Source: CAD feature listing. Evaluate the final solid. Frame: model axes, mm. A direction names the side the tool comes from. Give positions to 0.01 mm unless a question says otherwise; leave off trailing zeros. Write each loop counter-clockwise with the first axis right and the second up, starting at its lowest first coordinate (ties: lowest second). Pieces come first, ordered by that corner, then holes. Notation, with made-up numbers: (-22.75, 80.25) -> (30.25, 80.25) arc R13 ccw to (30.25, 99.25) -> close; hole circle Ø3 at (-32.75, -18.5). An arc over 180 degrees is marked (long way). Write item = value, one per line.
Autodesk Inventor part; units mm, degrees
ref_plane "YZ Plane" through (0, 0, 0) normal (1, 0, 0) x (0, 1, 0)
ref_plane "XZ Plane" through (0, 0, 0) normal (0, 1, 0) x (-1, 0, 0)
ref_plane "XY Plane" through (0, 0, 0) normal (0, 0, 1) x (1, 0, 0)
sketch "Эскиз1" plane through (0, 0, 0) normal (0, 0, 1) x (1, 0, 0)
  line L0 (0, 0) -> (58, 0)
  line L1 (58, 0) -> (58, 60)
  line L2 (58, 60) -> (0, 60)
  line L3 (0, 60) -> (0, 0)
  line L4 (0, 57) -> (58, 57) construction
  line L5 (0, 3) -> (58, 3) construction
  line L6 (3, 0) -> (3, 60) construction
  line L7 (55, 60) -> (55, 0) construction
  circle A0 centre (3, 57) radius 1.25
  circle A1 centre (55, 57) radius 1.25
  circle A2 centre (55, 3) radius 1.25
  circle A3 centre (3, 3) radius 1.25
  dimension "d0" = 58
  dimension "d1" = 60
  dimension "d2" = 52
  dimension "d3" = 54
  dimension "d4" = 3
  dimension "d5" = 3
  dimension "d6" = 2.5
extrude "Выдавливание1" add sketch "Эскиз1" along normal blind 1
sketch "Эскиз2" plane through (0, 0, 1) normal (0, 0, 1) x (1, 0, 0)
  line L0 (37, -2) -> (47, -2)
  line L1 (47, -2) -> (47, 10)
  line L2 (47, 10) -> (37, 10)
  line L3 (37, 10) -> (37, -2)
  line L4 (0, 60) -> (0, 0)
  line L5 (58, 0) -> (58, 60)
  line L6 (0, 0) -> (58, 0)
  dimension "d9" = 37
  dimension "d10" = 11
  dimension "d14" = 2
  dimension "d15" = 12
extrude "Выдавливание2" add sketch "Эскиз2" along normal blind 11
sketch "Эскиз3" plane through (0, 0, 1) normal (0, 0, 1) x (1, 0, 0)
  line L0 (7, 60) -> (19.5, 60)
  line L1 (19.5, 60) -> (19.5, 53)
  line L2 (19.5, 53) -> (7, 53)
  line L3 (7, 53) -> (7, 60)
  line L4 (58, 60) -> (0, 60)
  line L5 (0, 60) -> (0, 0)
  line L6 (58, 0) -> (58, 60)
  line L7 (30.5, 60) -> (43, 60)
  line L8 (43, 60) -> (43, 53)
  line L9 (43, 53) -> (30.5, 53)
  line L10 (30.5, 53) -> (30.5, 60)
  dimension "d16" = 7
  dimension "d18" = 15
  dimension "d19" = 12.5
  dimension "d20" = 7
extrude "Выдавливание3" add sketch "Эскиз3" along normal blind 6
sketch "Эскиз4" plane through (0, 0, 1) normal (0, 0, 1) x (1, 0, 0)
  line L0 (3, 50) -> (47, 50)
  line L1 (47, 50) -> (47, 35)
  line L2 (47, 35) -> (3, 35)
  line L3 (3, 35) -> (3, 50)
  line L4 (0, 60) -> (0, 0)
  line L5 (30.5, 60) -> (19.5, 60)
  dimension "d23" = 15
  dimension "d24" = 44
  dimension "d25" = 3
  dimension "d26" = 10
extrude "Выдавливание4" add sketch "Эскиз4" along normal blind 26
sketch "Эскиз5" plane through (0, 0, 1) normal (0, 0, 1) x (1, 0, 0)
  line L0 (3, 33) -> (46, 33)
  line L1 (46, 33) -> (46, 15)
  line L2 (46, 15) -> (3, 15)
  line L3 (3, 15) -> (3, 33)
  line L4 (0, 0) -> (37, 0)
  line L5 (0, 60) -> (0, 0)
  line L6 (58, 0) -> (58, 60)
  dimension "d29" = 15
  dimension "d30" = 3
  dimension "d31" = 18
  dimension "d32" = 12
extrude "Выдавливание5" add sketch "Эскиз5" along normal blind 17
sketch "Эскиз6" plane through (0, 0, 1) normal (0, 0, 1) x (1, 0, 0)
  line L0 (24, 12) -> (3, 12)
  line L1 (3, 12) -> (3, 6)
  line L2 (3, 6) -> (24, 6)
  line L3 (24, 6) -> (24, 12)
  line L4 (0, 0) -> (37, 0)
  line L5 (0, 60) -> (0, 0)
  dimension "d35" = 6
  dimension "d36" = 3
  dimension "d37" = 6
  dimension "d38" = 21
extrude "Выдавливание6" add sketch "Эскиз6" along normal blind 11
properties part number "Плата"
(1) Section query A-A (y = 3). Return loops of the section in (x, z), plus the area to 3 significant figures.
Values follow:
outline = (0, 0) -> (1.75, 0) -> (1.75, 1) -> (0, 1) -> close; (4.25, 0) -> (53.75, 0) -> (53.75, 1) -> (47, 1) -> (47, 12) -> (37, 12) -> (37, 1) -> (4.25, 1) -> close; (56.25, 0) -> (58, 0) -> (58, 1) -> (56.25, 1) -> close
area = 163 mm2
(2) Material intervals for line 1 (Y direction, x = 14, z = 1.5); line 2 (Y direction, x = 3, z = 0.4); line 3 (Y direction, x = 17, z = 9), sorted ascending.
Values follow:
line_1 = 6 to 12, 15 to 33, 35 to 50, 53 to 60
line_2 = 0 to 1.75, 4.25 to 55.75, 58.25 to 60
line_3 = 6 to 12, 15 to 33, 35 to 50
(3) First-contact query: pin 1 (5 mm diameter, centred on y = 8, z = 4, fed in from +X); pin 2 (12 mm diameter, centred on y = 34.5, z = 17.5, fed in from -X); pin 3 (2 mm diameter, centred on x = 39.5, z = 18, fed in from +Y); pin 4 (3 mm diameter, centred on x = 27, y = 7.5, fed in from -Z). Flat tips, straight axial feed; report the tip coordinate or a pass-through.
Values follow:
pin_1 = 47
pin_2 = 3
pin_3 = 50
pin_4 = 0
(4) Pull-direction query (Y, two-part tool) for faces 1 (the face through (42, -2, 6)), 2 (the face through (19.5, 57, 4)), 3 (the face through (56.19, 56.62, 0.49)); classes: pulls with the +Y half, pulls with the -Y half, needs draft (parallel to the pull), parting line crosses it, or undercut.
Values follow:
face_1 = pulls with the -Y half
face_2 = needs draft
face_3 = undercut
(5) Access query for faces 4 (the face through (37, 4, 6)), 5 (the face through (3, 24, 9)), 6 (the face through (43, 57, 4)), 7 (the face through (7, 56, 4)). Directions: +Z, -Z, +X, -X, +Y, -Y. A direction counts if a zero-diameter tool reaches every point of the face in a straight line with its end or side. Return the directions, or none.
Values follow:
face_4 = +Z, -Y
face_5 = +Z, -X, +Y, -Y
face_6 = +Z, +X, +Y
face_7 = +Z, -X, +Y
(6) Section query C-C (z = 14.5). Return loops of the section in (x, y).
Values follow:
outline = (3, 15) -> (46, 15) -> (46, 33) -> (3, 33) -> close; (3, 35) -> (47, 35) -> (47, 50) -> (3, 50) -> close
(7) Section query D-D (x = 18.5). Return loops of the section in (y, z).
Values follow:
outline = (0, 0) -> (60, 0) -> (60, 7) -> (53, 7) -> (53, 1) -> (50, 1) -> (50, 27) -> (35, 27) -> (35, 1) -> (33, 1) -> (33, 18) -> (15, 18) -> (15, 1) -> (12, 1) -> (12, 12) -> (6, 12) -> (6, 1) -> (0, 1) -> close
(8) Section query B-B (x = 55). Return loops of the section in (y, z), plus the area to 3 significant figures.
Values follow:
outline = (0, 0) -> (1.75, 0) -> (1.75, 1) -> (0, 1) -> close; (4.25, 0) -> (55.75, 0) -> (55.75, 1) -> (4.25, 1) -> close; (58.25, 0) -> (60, 0) -> (60, 1) -> (58.25, 1) -> close
area = 55.0 mm2
